CAD build for the part. Positions are in the model's coordinates, mm. A direction names the side the tool comes from. Round coordinates to 2 decimals unless told otherwise and drop trailing zeros. Write each loop counter-clockwise with the first axis right and the second up, starting at its lowest first coordinate (ties: lowest second). Pieces come first, ordered by that corner, then holes. Notation, with made-up numbers: (-18.5, -15) - (0.5, -15) arc R17 cw to (0.5, 0) - close; hole circle Ø11 at (62.5, 8.5). An arc over 180 degrees is marked (long way). Use one line per item in the form item = value. Start each with the question number.
Item 1: Drill centre lines: L1, parallel to X at y = 0, z = 4.25; L2, parallel to Z at x = 20.25, y = 0; L3, parallel to Z at x = 2.5, y = 5.75. Where is each one in solid material? Low to high.
Item 2: Band-saw the part on D-D, the plane y = -2.5. Give the number of separate pieces and of enclosed holes in the cut face, and give its area (3 significant figures).
Item 3: Tool access for faces 4 (the flat face through (12, -6.35, 0)), 5 (the flat face through (11.125, 5, 0)): list every direction of +Z, -Z, +X, -X, +Y, -Y with a clear straight run to the whole face (end or side of a thin tool).
Item 4: Band-saw the part on C-C, the plane x = 16.5. List the corners of the cut face in (y, z), and give its area (3 significant figures).
Item 5: Pin check, flat tips, straight feed: pin 1 (4 mm diameter, centred on y = 0, z = 0, fed in from +X); pin 2 (5 mm diameter, centred on y = 0, z = 1, fed in from -X); pin 3 (3 mm diameter, centred on y = -4.5, z = 0.5, fed in from -X). Stop position of each tip, or through.
Item 6: Band-saw the part on A-A, the plane x = 10.5. List the corners of the cut face in (y, z), and give its area (3 significant figures).
Item 7: Pull direction Z, two halves, no side cores. Call faces 1 (the flat face through (-6.35, 0, -5)), 2 (the flat face through (4, 0, -3.334)), 3 (the flat face through (9, 0, 6.35)): +Z half, -Z half, draft (parallel to the pull), parting line (faces both ways), or undercut.
Item 8: Band-saw the part on B-B, the plane x = 0. List the corners of the cut face in (y, z), and give its area (3 significant figures).
Autodesk Inventor part; units mm, degrees
ref_plane "dummy_XY" through (0, 0, 0) normal (0, 0, 1) x (1, 0, 0)
ref_plane "dummy_YZ" through (0, 0, 0) normal (1, 0, 0) x (0, 1, 0)
ref_plane "dummy_ZX" through (0, 0, 0) normal (0, 1, 0) x (0, 0, 1)
sketch "Sketch_1" plane through (0, 0, 0) normal (0, 0, 1) x (1, 0, 0)
  line L0 (-6.35, -6.35) -> (23.8252, -6.35)
  line L1 (23.8252, -6.35) -> (23.8252, 6.35)
  line L2 (23.8252, 6.35) -> (-6.35, 6.35)
  line L3 (-6.35, 6.35) -> (-6.35, -6.35)
extrude "Extrusion1" add sketch "Sketch_1" along normal mid plane 12.7
sketch "Sketch_2" plane through (0, 0, 0) normal (0, 1, 0) x (-1, 0, 0)
  line L0 (6.35, 3.3338) -> (-11.1252, 3.3338)
  line L1 (-11.1252, 3.3338) -> (-11.1252, -3.3338)
  line L2 (-11.1252, -3.3338) -> (6.35, -3.3338)
  line L3 (6.35, -3.3338) -> (6.35, 3.3338)
extrude "Extrusion2" cut sketch "Sketch_2" along normal mid plane 12.7
sketch "Sketch_3" plane through (0, 0, 0) normal (0, 0, 1) x (1, 0, 0)
  line L0 (23.8252, 0) -> (12.6492, 0)
  line L1 (12.6492, 0) -> (12.6492, 3.396)
  line L2 (12.6492, 3.396) -> (23.2524, 3.396)
  line L3 (23.2524, 3.396) -> (23.8252, 3.9688)
  line L4 (23.8252, 3.9688) -> (23.8252, 0)
  line L5 (23.8252, 0) -> (12.6492, 0)
revolve "Revolution1" cut sketch "Sketch_3" angle 360 about axis through (23.8252, 0, 0) along (1, 0, 0)
thread "Thread1"
sketch "Sketch5" plane through (12.6492, 0, 0) normal (1, 0, 0) x (0, 0, -1)
  point P0 (0, 0)
hole "Hole1" at (12.6492, 0, 0) direction (-1, 0, 0) diameter 6.792 depth 1.524
sketch "Sketch_5" plane through (0, 0, 0) normal (1, 0, 0) x (0, 1, 0)
  line L0 (0, -6.35) -> (0, 6.35)
  line L1 (0, 6.35) -> (4.3371, 6.35)
  line L2 (4.3371, 6.35) -> (3.194, 5.207)
  line L3 (3.194, 5.207) -> (3.194, -5.207)
  line L4 (3.194, -5.207) -> (4.3371, -6.35)
  line L5 (4.3371, -6.35) -> (0, -6.35)
  line L6 (0, -6.35) -> (0, 6.35)
revolve "Revolution2" cut sketch "Sketch_5" angle 360 about axis through (0, 0, -6.35) along (0, 0, -1)
sketch "Sketch_9" plane through (0, 0, 0) normal (0, 0, 1) x (1, 0, 0)
  line L0 (30.1752, 0) -> (23.8252, 0)
  line L1 (23.8252, 0) -> (23.8252, 6.35)
  arc A0 (23.8252, 6.35) -> (21.2852, 12.7) centre (6.6802, 3.175) ccw
  line L2 (21.2852, 12.7) -> (30.1752, 12.7)
  line L3 (30.1752, 12.7) -> (30.1752, 0)
  line L4 (30.1752, 0) -> (23.8252, 0)
revolve "Revolution3" cut sketch "Sketch_9" angle 360 about axis through (30.1752, 0, 0) along (1, 0, 0)
sketch "Sketch_10" plane through (0, 0, 0) normal (0, 0, 1) x (1, 0, 0)
  line L0 (-6.35, 0) -> (-12.7, 0)
  line L1 (-12.7, 0) -> (-12.7, 12.7)
  line L2 (-12.7, 12.7) -> (-3.81, 12.7)
  arc A0 (-3.81, 12.7) -> (-6.35, 6.35) centre (10.795, 3.175) ccw
  line L3 (-6.35, 6.35) -> (-6.35, 0)
  line L4 (-6.35, 0) -> (-12.7, 0)
revolve "Revolution4" cut sketch "Sketch_10" angle 360 about axis through (-6.35, 0, 0) along (1, 0, 0)
ref_plane "dummy_XY" through (0, 0, 0) normal (0, 0, 1) x (1, 0, 0)
ref_plane "dummy_YZ" through (0, 0, 0) normal (1, 0, 0) x (0, 1, 0)
ref_plane "dummy_ZX" through (0, 0, 0) normal (0, 1, 0) x (0, 0, 1)
ref_plane "h1_XY" through (-6.35, 6.35, 0) normal (0, 0, 1) x (1, 0, 0)
ref_plane "h1_YZ" through (-6.35, 6.35, 0) normal (1, 0, 0) x (0, 1, 0)
ref_plane "h1_ZX" through (-6.35, 6.35, 0) normal (0, 1, 0) x (0, 0, 1)
ref_plane "h2_XY" through (-6.35, -6.35, 0) normal (0, 0, 1) x (1, 0, 0)
ref_plane "h2_YZ" through (-6.35, -6.35, 0) normal (1, 0, 0) x (0, 1, 0)
ref_plane "h2_ZX" through (-6.35, -6.35, 0) normal (0, 1, 0) x (0, 0, 1)
ref_plane "l1_XY" through (23.8252, 6.35, 0) normal (0, 0, 1) x (1, 0, 0)
ref_plane "l1_YZ" through (23.8252, 6.35, 0) normal (1, 0, 0) x (0, 1, 0)
ref_plane "l1_ZX" through (23.8252, 6.35, 0) normal (0, 1, 0) x (0, 0, 1)
ref_plane "l11_XY" through (23.8252, 6.35, 0) normal (0, 0, 1) x (1, 0, 0)
ref_plane "l11_YZ" through (23.8252, 6.35, 0) normal (1, 0, 0) x (0, 1, 0)
ref_plane "l11_ZX" through (23.8252, 6.35, 0) normal (0, 1, 0) x (0, 0, 1)
ref_plane "l12_XY" through (0, 6.35, 0) normal (0, 0, 1) x (1, 0, 0)
ref_plane "l12_YZ" through (0, 6.35, 0) normal (1, 0, 0) x (0, 1, 0)
ref_plane "l12_ZX" through (0, 6.35, 0) normal (0, 1, 0) x (0, 0, 1)
ref_plane "l2_XY" through (-6.35, 6.35, 0) normal (0, 0, 1) x (1, 0, 0)
ref_plane "l2_YZ" through (-6.35, 6.35, 0) normal (1, 0, 0) x (0, 1, 0)
ref_plane "l2_ZX" through (-6.35, 6.35, 0) normal (0, 1, 0) x (0, 0, 1)
ref_plane "l21_XY" through (23.8252, 0, 0) normal (0, 1, 0) x (1, 0, 0)
ref_plane "l21_YZ" through (23.8252, 0, 0) normal (1, 0, 0) x (0, 0, -1)
ref_plane "l21_ZX" through (23.8252, 0, 0) normal (0, 0, -1) x (0, 1, 0)
ref_plane "l22_XY" through (11.1252, 0, 0) normal (0, 1, 0) x (1, 0, 0)
ref_plane "l22_YZ" through (11.1252, 0, 0) normal (1, 0, 0) x (0, 0, -1)
ref_plane "l22_ZX" through (11.1252, 0, 0) normal (0, 0, -1) x (0, 1, 0)
ref_plane "piston_rod_clevis_XY" through (23.8252, 0, 0) normal (1, 0, 0) x (0, 0, -1)
ref_plane "piston_rod_clevis_YZ" through (23.8252, 0, 0) normal (0, 0, -1) x (0, 1, 0)
ref_plane "piston_rod_clevis_ZX" through (23.8252, 0, 0) normal (0, 1, 0) x (1, 0, 0)
ref_plane "rod_clevis_body_XY" through (0, 0, 0) normal (0, 0, 1) x (1, 0, 0)
ref_plane "rod_clevis_body_YZ" through (0, 0, 0) normal (1, 0, 0) x (0, 1, 0)
ref_plane "rod_clevis_body_ZX" through (0, 0, 0) normal (0, 1, 0) x (0, 0, 1)
ref_plane "th1_XY" through (23.8252, 3.9688, 0) normal (0, 0, 1) x (1, 0, 0)
ref_plane "th1_YZ" through (23.8252, 3.9688, 0) normal (1, 0, 0) x (0, 1, 0)
ref_plane "th1_ZX" through (23.8252, 3.9688, 0) normal (0, 1, 0) x (0, 0, 1)
ref_plane "th2_XY" through (23.8252, -3.9688, 0) normal (0, 0, 1) x (1, 0, 0)
ref_plane "th2_YZ" through (23.8252, -3.9688, 0) normal (1, 0, 0) x (0, 1, 0)
ref_plane "th2_ZX" through (23.8252, -3.9688, 0) normal (0, 1, 0) x (0, 0, 1)
ref_plane "to_cylinder_XY" through (11.1252, 0, 0) normal (1, 0, 0) x (0, 0, -1)
ref_plane "to_cylinder_YZ" through (11.1252, 0, 0) normal (0, 0, -1) x (0, 1, 0)
ref_plane "to_cylinder_ZX" through (11.1252, 0, 0) normal (0, 1, 0) x (1, 0, 0)
ref_plane "w1_XY" through (23.8252, 0, -6.35) normal (0, 1, 0) x (1, 0, 0)
ref_plane "w1_YZ" through (23.8252, 0, -6.35) normal (1, 0, 0) x (0, 0, -1)
ref_plane "w1_ZX" through (23.8252, 0, -6.35) normal (0, 0, -1) x (0, 1, 0)
ref_plane "w11_XY" through (-6.35, 0, -3.3338) normal (0, 1, 0) x (1, 0, 0)
ref_plane "w11_YZ" through (-6.35, 0, -3.3338) normal (1, 0, 0) x (0, 0, -1)
ref_plane "w11_ZX" through (-6.35, 0, -3.3338) normal (0, 0, -1) x (0, 1, 0)
ref_plane "w12_XY" through (-6.35, 0, 3.3338) normal (0, 1, 0) x (1, 0, 0)
ref_plane "w12_YZ" through (-6.35, 0, 3.3338) normal (1, 0, 0) x (0, 0, -1)
ref_plane "w12_ZX" through (-6.35, 0, 3.3338) normal (0, 0, -1) x (0, 1, 0)
ref_plane "w2_XY" through (23.8252, 0, 6.35) normal (0, 1, 0) x (1, 0, 0)
ref_plane "w2_YZ" through (23.8252, 0, 6.35) normal (1, 0, 0) x (0, 0, -1)
ref_plane "w2_ZX" through (23.8252, 0, 6.35) normal (0, 0, -1) x (0, 1, 0)
properties part number "D-14059"
Determined:
q1.L1 = -6.35 to -3.19, 3.19 to 23.83
q1.L2 = -6.35 to -3.4, 3.4 to 6.35
q1.L3 = -6.35 to -3.33, 3.33 to 6.35
q2.separate_pieces = 4
q2.enclosed_holes = 0
q2.area = 180 mm²
q3.face_4 = +Z, -Z, +X, -X, -Y
q3.face_5 = -X, +Y, -Y
q4.outline = (-6.35, -6.35) - (6.35, -6.35) - (6.35, 6.35) - (-6.35, 6.35) - close; hole circle Ø6.79 at (0, 0)
q4.area = 125 mm²
q5.pin_1 = through
q5.pin_2 = -6.35
q5.pin_3 = 11.13
q6.outline = (-6.35, -6.35) - (6.35, -6.35) - (6.35, -3.33) - (-6.35, -3.33) - close; (-6.35, 3.33) - (6.35, 3.33) - (6.35, 6.35) - (-6.35, 6.35) - close
q6.area = 76.6 mm²
q7.face_1 = draft
q7.face_2 = undercut
q7.face_3 = +Z half
q8.outline = (-6.35, -6.35) - (-4.34, -6.35) - (-3.19, -5.21) - (-3.19, -3.33) - (-6.35, -3.33) - close; (-6.35, 3.33) - (-3.19, 3.33) - (-3.19, 5.21) - (-4.34, 6.35) - (-6.35, 6.35) - close; (3.19, -5.21) - (4.34, -6.35) - (6.35, -6.35) - (6.35, -3.33) - (3.19, -3.33) - close; (3.19, 3.33) - (6.35, 3.33) - (6.35, 6.35) - (4.34, 6.35) - (3.19, 5.21) - close
q8.area = 35.5 mm²
